Could you check a few things on this model? Use its own coordinates, in mm. A direction names the side the tool comes from. Coordinates: 2 decimals unless noted, no trailing zeros. Order: outer loops, then holes, each group sorted by start corner. A loop starts at its lowest first (then second) coordinate and runs counter-clockwise, first axis right, second up. Notation, with made-up numbers: M 52,2 L 105,2 A22 ccw 105,17 Z; hole C 51,4.5 d5. An arc over 180 degrees is marked long. One line per question, with ' | ' between items. Start each with the question number.
Autodesk Inventor part; units mm, degrees
ref_plane "YZ Plane" through (0, 0, 0) normal (1, 0, 0) x (0, 1, 0)
ref_plane "XZ Plane" through (0, 0, 0) normal (0, 1, 0) x (-1, 0, 0)
ref_plane "XY Plane" through (0, 0, 0) normal (0, 0, 1) x (1, 0, 0)
sketch "Sketch1" plane through (0, 0, 0) normal (0, 1, 0) x (-1, 0, 0)
  line L0 (0, 0) -> (-100, 0)
  line L1 (-100, 0) -> (-100, -88)
  line L2 (-100, -88) -> (0, -88)
  line L3 (0, -88) -> (0, 0)
  line L4 (-9, -23.5) -> (-32, -23.5)
  line L5 (-33, -22.5) -> (-33, -13.5)
  line L6 (-32, -12.5) -> (-9, -12.5)
  line L7 (-8, -13.5) -> (-8, -22.5)
  arc A0 (-9, -23.5) -> (-8, -22.5) centre (-9, -22.5) ccw
  arc A1 (-8, -13.5) -> (-9, -12.5) centre (-9, -13.5) ccw
  arc A2 (-32, -12.5) -> (-33, -13.5) centre (-32, -13.5) ccw
  arc A3 (-33, -22.5) -> (-32, -23.5) centre (-32, -22.5) ccw
  line L8 (-9, -77.5) -> (-32, -77.5)
  line L9 (-33, -76.5) -> (-33, -67.5)
  line L10 (-32, -66.5) -> (-9, -66.5)
  line L11 (-8, -67.5) -> (-8, -76.5)
  arc A4 (-9, -77.5) -> (-8, -76.5) centre (-9, -76.5) ccw
  arc A5 (-8, -67.5) -> (-9, -66.5) centre (-9, -67.5) ccw
  arc A6 (-32, -66.5) -> (-33, -67.5) centre (-32, -67.5) ccw
  arc A7 (-33, -76.5) -> (-32, -77.5) centre (-32, -76.5) ccw
  line L12 (-68, -77.5) -> (-91, -77.5)
  line L13 (-92, -76.5) -> (-92, -67.5)
  line L14 (-91, -66.5) -> (-68, -66.5)
  line L15 (-67, -67.5) -> (-67, -76.5)
  arc A8 (-68, -77.5) -> (-67, -76.5) centre (-68, -76.5) ccw
  arc A9 (-67, -67.5) -> (-68, -66.5) centre (-68, -67.5) ccw
  arc A10 (-91, -66.5) -> (-92, -67.5) centre (-91, -67.5) ccw
  arc A11 (-92, -76.5) -> (-91, -77.5) centre (-91, -76.5) ccw
  line L16 (-68, -23.5) -> (-91, -23.5)
  line L17 (-92, -22.5) -> (-92, -13.5)
  line L18 (-91, -12.5) -> (-68, -12.5)
  line L19 (-67, -13.5) -> (-67, -22.5)
  arc A12 (-68, -23.5) -> (-67, -22.5) centre (-68, -22.5) ccw
  arc A13 (-67, -13.5) -> (-68, -12.5) centre (-68, -13.5) ccw
  arc A14 (-91, -12.5) -> (-92, -13.5) centre (-91, -13.5) ccw
  arc A15 (-92, -22.5) -> (-91, -23.5) centre (-91, -22.5) ccw
  line L20 (-8, -72) -> (-92, -72) construction
  line L21 (-92, -18) -> (-8, -18) construction
  point P0 (-50, -18)
  point P1 (-50, 0)
  dimension "d0" = 100
  dimension "d1" = 88
  dimension "d2" = 1
  dimension "d3" = 25
  dimension "d4" = 11
  dimension "d5" = 1
  dimension "d6" = 25
  dimension "d7" = 11
  dimension "d8" = 1
  dimension "d9" = 25
  dimension "d10" = 11
  dimension "d11" = 1
  dimension "d12" = 25
  dimension "d13" = 11
  dimension "d14" = 54
  dimension "d15" = 18
  dimension "d16" = 8
extrude "Extrusion1" add sketch "Sketch1" along normal blind 6.5
chamfer "Chamfer1" distance 4 angle 45 4 edges at (0, 3.25, 0) (100, 3.25, 0) (100, 3.25, -88) (0, 3.25, -88)
sketch "Sketch2" plane through (0, 6.5, 0) normal (0, 1, 0) x (1, 0, 0)
  line L0 (4, 0) -> (96, 0)
  line L1 (9.5, 44) -> (17.5, 44)
  line L2 (17.5, 44) -> (17.5, 37.5)
  line L3 (17.5, 37.5) -> (9.5, 37.5)
  line L4 (9.5, 37.5) -> (9.5, 44)
  line L5 (32.5, 44) -> (40.5, 44)
  line L6 (40.5, 44) -> (40.5, 37.5)
  line L7 (40.5, 37.5) -> (32.5, 37.5)
  line L8 (32.5, 37.5) -> (32.5, 44)
  line L9 (59.5, 44) -> (67.5, 44)
  line L10 (67.5, 44) -> (67.5, 37.5)
  line L11 (67.5, 37.5) -> (59.5, 37.5)
  line L12 (59.5, 37.5) -> (59.5, 44)
  line L13 (82.5, 44) -> (90.5, 44)
  line L14 (90.5, 44) -> (90.5, 37.5)
  line L15 (90.5, 37.5) -> (82.5, 37.5)
  line L16 (82.5, 37.5) -> (82.5, 44)
  line L17 (17.5, 44) -> (32.5, 37.5) construction
  line L18 (32.5, 44) -> (17.5, 37.5) construction
  line L19 (67.5, 37.5) -> (82.5, 44) construction
  line L20 (82.5, 37.5) -> (67.5, 44) construction
  circle A0 centre (25, 40.75) radius 2.25
  circle A1 centre (75, 40.75) radius 2.25
  line L21 (40.5, 40.75) -> (59.5, 40.75) construction
  point P0 (0, 0)
  point P1 (50, 40.75)
  point P2 (50, 0)
  dimension "d22" = 6.5
  dimension "d23" = 8
  dimension "d24" = 15
  dimension "d25" = 15
  dimension "d26" = 4.5
  dimension "d27" = 4.5
  dimension "d28" = 50
  dimension "d29" = 37.5
extrude "Extrusion2" cut sketch "Sketch2" against normal through all
sketch "Sketch3" plane through (0, 6.5, 0) normal (0, 1, 0) x (1, 0, 0)
  line L0 (9, 77.5) -> (32, 77.5)
  line L1 (8, 67.5) -> (8, 76.5)
  line L2 (32, 12.5) -> (9, 12.5)
  line L3 (0, 84) -> (0, 4)
  line L4 (4, 0) -> (96, 0)
  line L5 (100, 4) -> (100, 84)
  line L6 (5, 81.75) -> (95, 81.75) construction
  line L7 (95, 81.75) -> (95, 8.25) construction
  line L8 (95, 8.25) -> (5, 8.25) construction
  line L9 (5, 8.25) -> (5, 81.75) construction
  circle A0 centre (5, 81.75) radius 4.5 construction
  circle A1 centre (95, 81.75) radius 4.5 construction
  circle A2 centre (95, 8.25) radius 4.5 construction
  circle A3 centre (5, 8.25) radius 4.5 construction
  circle A4 centre (5, 81.75) radius 2.25
  circle A5 centre (95, 81.75) radius 2.25
  circle A6 centre (95, 8.25) radius 2.25
  circle A7 centre (5, 8.25) radius 2.25
  point P0 (0, 0)
  dimension "d32" = 9
  dimension "d33" = 4.5
  dimension "d34" = 8
  dimension "d35" = 12.5
  dimension "d36" = 5
  dimension "d37" = 5
  dimension "d38" = 8.25
  dimension "d39" = 4.25
extrude "Extrusion3" cut sketch "Sketch3" against normal through all
sketch "Sketch4" plane through (0, 6.5, 0) normal (0, 1, 0) x (1, 0, 0)
  line L0 (4, 0) -> (96, 0)
  line L1 (96, 88) -> (4, 88)
  circle A0 centre (37.5, 11.75) radius 2.25
  circle A1 centre (62.5, 11.75) radius 2.25
  line L2 (37.5, 11.75) -> (62.5, 11.75) construction
  point P0 (0, 0)
  point P1 (50, 11.75)
  point P2 (50, 0)
  dimension "d42" = 4.5
  dimension "d43" = 25
  dimension "d44" = 11.75
extrude "Extrusion4" cut sketch "Sketch4" against normal through all
sketch "Sketch5" plane through (0, 6.5, 0) normal (0, 1, 0) x (1, 0, 0)
  line L0 (32.5, 44) -> (40.5, 44)
  line L1 (96, 88) -> (4, 88)
  circle A0 centre (50, 63.75) radius 2.25
  point P0 (0, 0)
  point P1 (50, 88)
  dimension "d47" = 4.5
  dimension "d48" = 19.75
extrude "Extrusion5" cut sketch "Sketch5" against normal through all
equation "\"d25\" = d24"
equation "\"d37\" = d36"
equation "\"d39\" = d35 - d38"
properties part number "x_carryage_back" material "Plywood, Finish"
(1) Imagine slicing it at A-A, the plane x = 25. Write out the boundary of the cut face in (y, z).
(2) Imagine slicing it at B-B, the plane z = -63.75. Write out the boundary of the cut face in (x, y), plus the area to 3 significant figures.
(3) Imagine slicing it at C-C, the plane x = 62.5. Write out the boundary of the cut face in (y, z), plus the area to 4 significant figures.
(4) We'd pull the mould along Z, two halves only. Please class faces 1 (the flat face through (51, 6.5, -43)), 2 (the flat face through (92, 3, -18)), 3 (the flat face through (2, 3, -2)): +Z half, -Z half, draft (parallel to the pull), parting line (faces both ways), or undercut.
(5) If I drill on line 1 along Z through (x, y) = (27.5, 2); line 2 along X through (y, z) = (4.5, -11.75); line 3 along Z through (x, y) = (25, 4.25), over which ranges is the centre line in solid material (lowest first)? Write a range as from..to.
(6) On a 3-axis mill with a long thin cutter (end or side, diameter ignored), from which of +Z, -Z, +X, -X, +Y, -Y can I reach the whole of each face in a straight line? I mean faces 4 (the flat face through (80, 3, -12.5)), 5 (the flat face through (51, 0, -43)). Say none if no direction works.
(7) Imagine slicing it at D-D, the plane z = -81.75. Write out the boundary of the cut face in (x, y), plus the area to 4 significant figures.
Answers:
1) outline: M 0,-88 L 6.5,-88 L 6.5,-77.5 L 0,-77.5 Z; M 0,-66.5 L 6.5,-66.5 L 6.5,-43 L 0,-43 Z; M 0,-38.5 L 6.5,-38.5 L 6.5,-23.5 L 0,-23.5 Z; M 0,-12.5 L 6.5,-12.5 L 6.5,0 L 0,0 Z
2) outline: M 0,0 L 47.75,0 L 47.75,6.5 L 0,6.5 Z; M 52.25,0 L 100,0 L 100,6.5 L 52.25,6.5 Z | area: 621 mm²
3) outline: M 0,-88 L 6.5,-88 L 6.5,-44 L 0,-44 Z; M 0,-37.5 L 6.5,-37.5 L 6.5,-14 L 0,-14 Z; M 0,-9.5 L 6.5,-9.5 L 6.5,0 L 0,0 Z | area: 500.5 mm²
4) face 1: draft | face 2: undercut | face 3: +Z half
5) line 1: -88..-77.5, -66.5..-23.5, -12.5..0 | line 2: 0..35.25, 39.75..60.25, 64.75..100 | line 3: -88..-77.5, -66.5..-43, -38.5..-23.5, -12.5..0
6) face 4: +Y, -Y | face 5: +Z, -Z, +X, -X, -Y
7) outline: M 0,0 L 2.75,0 L 2.75,6.5 L 0,6.5 Z; M 7.25,0 L 92.75,0 L 92.75,6.5 L 7.25,6.5 Z; M 97.25,0 L 100,0 L 100,6.5 L 97.25,6.5 Z | area: 591.5 mm²
